The listing builds one solid part. Answer for the finished solid, in the listing's coordinates (mm). Face numbers are marked on the shaded views. A direction names the side the tool comes from. Give positions to 0.01 mm unless a question says otherwise; leave off trailing zeros. Write each loop counter-clockwise with the first axis right and the second up, starting at its lowest first coordinate (ties: lowest second). Pieces come first, ordered by that corner, then holes. Notation, with made-up numbers: (-9, -13) - (17, -13) arc R24 ccw to (17, 16) - close; hole circle Ø2 at (25, 76.25). An arc over 180 degrees is marked (long way). Answer as CSV lines item,"result". Start each with the question number.
(1) Straight lines are drawn through the part: probe 1 along Y at (x, z) = (0, 46.5); probe 2 along Y at (x, z) = (0, 10); probe 3 along X at (y, z) = (0.5, 14.5). For each, find the intervals that lie inside material, in ascending order.
(2) For the marked faces 1 and 2, determine the directions among +Z, -Z, +X, -X, +Y, -Y from which every point of the face is accessible in a straight line to the end or side of a thin tool.
(3) Find section C-C (z = 32.5). Write down the section's boundary in (x, y), then the cut area to 3 significant figures.
(4) Find section D-D (z = 20). Write down the section's boundary in (x, y) (1 decimal), then the cut area to 3 significant figures.
(5) For a pull along X with two mould halves and no side action, classify the marked faces 3, 4 and 5 as pulls with the +X half, pulls with the -X half, needs draft (parallel to the pull), parting line crosses it, or undercut.
(6) Find section A-A (x = 0). Write down the section's boundary in (y, z).
(7) Each of these flat-tipped pins is pushed along its axis until it touches: pin 1 Ø3 at (x, y) = (-6.5, 3) entering from +Z; pin 2 Ø10 at (x, y) = (-16.5, 5) entering from -Z; pin 3 Ø4 at (y, z) = (3, 36) entering from -X; pin 4 Ø4 at (x, z) = (-13.5, 14) entering from -Y. Where does it stop, or does it pass through?
from build123d import *

# Parameters (mm, degrees)
CYLINDER2I_R     = 10.668
CYLINDER2I_DEPTH = 23.01875
CYLINDER1I_R     = 16.7005
CYLINDER1I_DEPTH = 23.01875
CYLINDER2_R      = 13.890625
CYLINDER2_DEPTH  = 21.03176
CYLINDER1_R      = 20.6375
CYLINDER1_DEPTH  = 25.00574


with BuildPart() as cone001:
    # Cone001 → Cone001 (revolve)
    with BuildSketch(Plane(origin=(0, 0, 23.01875), x_dir=(1, 0, 0), z_dir=(0, -1, 0))):
        Polygon((0, 0), (13.0683, 0), (7.6454, 10.31875), (0, 10.31875), align=None)
    revolve(axis=Axis((0, 0, 23.01875), (0, 0, 1)))


with BuildPart() as cylinder2i:
    # Cylinder2i → Cylinder2i (new body)
    with BuildSketch(Plane.XY.offset(33.3375)):
        Circle(CYLINDER2I_R)
    extrude(amount=CYLINDER2I_DEPTH)


with BuildPart() as innerparts:
    # Cylinder1i → Cylinder1i (new body)
    with BuildSketch(Plane.XY):
        Circle(CYLINDER1I_R)
    extrude(amount=CYLINDER1I_DEPTH)

    # InnerParts: union Cone001, Cylinder2i
    add(cone001.part)
    add(cylinder2i.part)


with BuildPart() as cone:
    # Cone → Cone (revolve)
    with BuildSketch(Plane(origin=(0, 0, 25.00574), x_dir=(1, 0, 0), z_dir=(0, -1, 0))):
        Polygon((0, 0), (20.6375, 0), (13.890625, 10.31875), (0, 10.31875), align=None)
    revolve(axis=Axis((0, 0, 25.00574), (0, 0, 1)))


with BuildPart() as cylinder2:
    # Cylinder2 → Cylinder2 (new body)
    with BuildSketch(Plane.XY.offset(35.32449)):
        Circle(CYLINDER2_R)
    extrude(amount=CYLINDER2_DEPTH)


with BuildPart() as coupling:
    # Cylinder1 → Cylinder1 (new body)
    with BuildSketch(Plane.XY):
        Circle(CYLINDER1_R)
    extrude(amount=CYLINDER1_DEPTH)

    # OuterParts: union Cone, Cylinder2
    add(cone.part)
    add(cylinder2.part)

    # coupling: cut InnerParts
    add(innerparts.part, mode=Mode.SUBTRACT)


solid = coupling.part
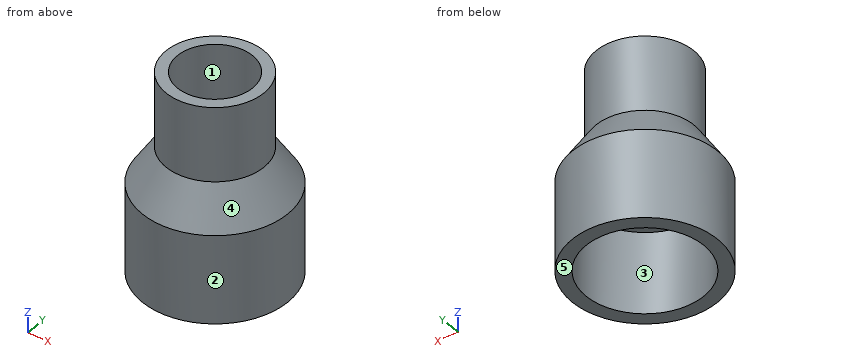
Result set:
1,probe 1,"-13.89 to -10.67, 10.67 to 13.89"
1,probe 2,"-20.64 to -16.7, 16.7 to 20.64"
1,probe 3,"-20.63 to -16.69, 16.69 to 20.63"
2,face 1,"+Z"
2,face 2,"+Z, -Z"
3,outline,"circle Ø31.47 at (0, 0); hole circle Ø16.17 at (0, 0)"
3,area,"573 mm^2"
4,outline,"circle Ø41.3 at (0, 0); hole circle Ø33.4 at (0, 0)"
4,area,"462 mm^2"
5,face 3,"undercut"
5,face 4,"parting line crosses it"
5,face 5,"needs draft"
6,outline,"(-20.64, 0) - (-16.7, 0) - (-16.7, 23.02) - (-13.07, 23.02) - (-7.65, 33.34) - (-10.67, 33.34) - (-10.67, 56.36) - (-13.89, 56.36) - (-13.89, 35.32) - (-20.64, 25.01) - close; (7.65, 33.34) - (13.07, 23.02) - (16.7, 23.02) - (16.7, 0) - (20.64, 0) - (20.64, 25.01) - (13.89, 35.32) - (13.89, 56.36) - (10.67, 56.36) - (10.67, 33.34) - close"
7,pin 1,"z = 33.34"
7,pin 2,"z = 0"
7,pin 3,"x = -14.5"
7,pin 4,"y = -17.14"
